Could you check a few things on this model? Use its own coordinates, in mm. A direction names the side the tool comes from. Give positions to 0.01 mm unless a question says otherwise; leave off trailing zeros. Order: outer loops, then holes, each group sorted by start corner. A loop starts at its lowest first (then second) coordinate and runs counter-clockwise, first axis right, second up. Notation, with made-up numbers: (7, -21.75) -> (30, -21.75) arc R24 cw to (30, 8.25) -> close; hole circle Ø5 at (32.25, 83). An arc over 180 degrees is marked (long way). One line per item, written item: value.
```python
from build123d import *

# Parameters (mm, degrees)
BOSS_EXTRUDE6_DEPTH = 76.2


with BuildPart() as part:
    # Sketch1 → Boss-Extrude6 (new body)
    with BuildSketch(Plane(origin=(0, 0, -3683), x_dir=(-1, 0, 0), z_dir=(0, 0, -1))):
        with BuildLine():
            Line((12.7, 4.064), (3.556, 4.064))
            ThreePointArc((3.556, 4.064), (3.106987194, 4.249987194), (2.921, 4.699))
            Line((2.921, 4.699), (2.921, 6.223))
            ThreePointArc((2.921, 6.223), (3.106987194, 6.672012806), (3.556, 6.858))
            Line((3.556, 6.858), (6.376363549, 6.858))
            Line((6.376363549, 6.858), (6.376363549, 7.365999958))
            Line((6.376363549, 7.365999958), (2.54, 11.938))
            Line((2.54, 11.938), (-2.54, 11.938))
            Line((-2.54, 11.938), (-6.376363549, 7.365999958))
            Line((-6.376363549, 7.365999958), (-6.376363549, 6.858))
            Line((-6.376363549, 6.858), (-3.556, 6.858))
            ThreePointArc((-3.556, 6.858), (-3.106987194, 6.672012806), (-2.921, 6.223))
            Line((-2.921, 6.223), (-2.921, 4.699))
            ThreePointArc((-2.921, 4.699), (-3.106987194, 4.249987194), (-3.556, 4.064))
            Line((-3.556, 4.064), (-12.7, 4.064))
            Line((-12.7, 4.064), (-12.7, 0))
            Line((-12.7, 0), (12.7, 0))
            Line((12.7, 0), (12.7, 4.064))
        make_face()
    extrude(amount=BOSS_EXTRUDE6_DEPTH)


solid = part.part
```
1) For faces 1 (the flat face through (0, 11.938, -3721)), 2 (the flat face through (-5, 6.858, -3721)), 3 (the flat face through (5, 6.858, -3721)), which set-ups out of +Z, -Z, +X, -X, +Y, -Y let a thin tool reach every point of the face, with its end or its side?
Answer below:
face 1: +Z, -Z, +X, -X, +Y
face 2: +Z, -Z, -X
face 3: +Z, -Z, +X
2) Suppose I cut it at C-C, the plane x = 10.5. Write out the boundary of the cut face in (y, z), then the cut area to 3 significant figures.
Answer below:
outline: (0, -3759.2) -> (4.06, -3759.2) -> (4.06, -3683) -> (0, -3683) -> close
area: 310 mm2
3) For P1, Ø5, axis at x = -9, y = 9.5, coming from the -Z side; P2, Ø10, axis at x = 8.5, z = -3702, coming from the +Y side; P3, Ø0.8, axis at y = 5, z = -3710, coming from the +X side; P4, Ø0.8, axis at y = 6, z = -3728, coming from the -X side, each with a flat end and sliding along its axis, tell me the tip position at first contact or that it passes through.
Answer below:
P1: passes through
P2: stops at y = 10.79
P3: stops at x = 2.93
P4: stops at x = -2.95
4) Suppose I cut it at B-B, the plane x = 5.25. Write out the boundary of the cut face in (y, z).
Answer below:
outline: (0, -3759.2) -> (4.06, -3759.2) -> (4.06, -3683) -> (0, -3683) -> close; (6.86, -3759.2) -> (8.71, -3759.2) -> (8.71, -3683) -> (6.86, -3683) -> close
5) We'd pull the mould along Y, two halves only. Please class faces 4 (the flat face through (-2.921, 5, -3721)), 5 (the flat face through (4.431, 9.684, -3720.567)), 6 (the flat face through (0, 5, -3683)): +Y half, -Y half, draft (parallel to the pull), parting line (faces both ways), or undercut.
Answer below:
face 4: undercut
face 5: +Y half
face 6: draft
6) Suppose I cut it at A-A, the plane z = -3733.5. Write out the boundary of the cut face in (x, y) (3 decimals).
Answer below:
outline: (-12.7, 0) -> (12.7, 0) -> (12.7, 4.064) -> (3.556, 4.064) arc R0.635 cw to (2.921, 4.699) -> (2.921, 6.223) arc R0.635 cw to (3.556, 6.858) -> (6.376, 6.858) -> (6.376, 7.366) -> (2.54, 11.938) -> (-2.54, 11.938) -> (-6.376, 7.366) -> (-6.376, 6.858) -> (-3.556, 6.858) arc R0.635 cw to (-2.921, 6.223) -> (-2.921, 4.699) arc R0.635 cw to (-3.556, 4.064) -> (-12.7, 4.064) -> close
7) If I drill on line 1 along X through (y, z) = (7, -3745.5); line 2 along Y through (x, z) = (-8.75, -3749.5); line 3 along Y through (x, z) = (6, -3726.5), over which ranges is the centre line in solid material (lowest first)?
Answer below:
line 1: x = -6.38 to 6.38
line 2: y = 0 to 4.06
line 3: y = 0 to 4.06, 6.86 to 7.81
